Autodesk Fusion 360 part; units mm, degrees
sketch "Sketch1" plane through (0, 0, 0) normal (0, 0, 1) x (1, 0, 0)
  line L0 (-4.125, 1.2) -> (4.125, 1.2)
  line L1 (4.125, 1.2) -> (4.125, -1.2)
  line L2 (4.125, -1.2) -> (-4.125, -1.2)
  line L3 (-4.125, -1.2) -> (-4.125, 1.2)
  line L4 (-4.125, 1.2) -> (4.125, -1.2) construction
  line L5 (4.125, 1.2) -> (-4.125, -1.2) construction
  circle A0 centre (-2.925, 0) radius 1.2
  circle A1 centre (2.925, 0) radius 1.2
  line L6 (-2.925, -0.8) -> (2.925, -0.8)
  arc A2 (2.925, -0.8) -> (2.925, 0.8) centre (2.925, 0) ccw
  line L7 (2.925, 0.8) -> (-2.925, 0.8)
  arc A3 (-2.925, 0.8) -> (-2.925, -0.8) centre (-2.925, 0) ccw
  line L8 (-2.925, 0) -> (2.925, 0) construction
  dimension "d1" = 8.25
  dimension "d2" = 2.4
  dimension "d3" = 0.4
extrude "Extrude1" add sketch "Sketch1" along normal blind 6.7 contours L0 A0 A1 L7 | A0 L6 L7 A3 | A1 L6 A2 L7 | L2 A0 A1 L6 picked at (-3.9868, -0.0769) picked at (3.9868, -0.0769)
sketch "Sketch2" plane through (0, 0, 6.7) normal (0, 0, 1) x (-1, 0, 0)
  arc A0 (2.925, -0.8) -> (2.925, 0.8) centre (2.925, 0) ccw
  line L0 (2.925, -0.8) -> (-2.925, -0.8)
  arc A1 (-2.925, 0.8) -> (-2.925, -0.8) centre (-2.925, 0) ccw
  line L1 (-2.925, 0.8) -> (2.925, 0.8)
  arc A2 (2.925, -1.2) -> (2.925, 1.2) centre (2.925, 0) ccw
  line L2 (2.925, 1.2) -> (-2.925, 1.2)
  arc A3 (-2.925, 1.2) -> (-2.925, -1.2) centre (-2.925, 0) ccw
  line L3 (-2.925, -1.2) -> (2.925, -1.2)
  line L4 (2.25, 3.5) -> (-2.25, 3.5)
  arc A4 (-2.25, 3.5) -> (-2.25, -3.5) centre (-2.25, 0) ccw
  line L5 (-2.25, -3.5) -> (2.25, -3.5)
  arc A5 (2.25, -3.5) -> (2.25, 3.5) centre (2.25, 0) ccw
  line L6 (2.25, 0) -> (-2.25, 0) construction
  line L7 (5.75, 0) -> (5.75, -5.6994) construction
  line L8 (-5.75, 0) -> (-5.75, -5.542) construction
  dimension "d7" = 7
  dimension "d8" = 11.5
extrude "Extrude2" add sketch "Sketch2" along normal blind 15.3 contours A0 L0 A1 L1 | A2 L2 A3 L3 | L4 A4 L5 A5
ref_plane "WorkPlane2" through (0, 0, 28.7) normal (0, 0, -1) x (1, 0, 0)
sketch "Sketch3" plane through (0, 0, 28.7) normal (0, 0, -1) x (-1, 0, 0)
  circle A0 centre (0, 0) radius 3.2
  dimension "d12" = 6.4
loft "Loft1" add profiles "Sketch3" section 1 face at (-0.75, 1.1667, 22) section 2
extrude "Extrude3" add sketch "Sketch3" against normal blind 6.3
fillet "Fillet1" radius 20 4 edges at (0.3491, 3.1809, 28.7) (3.1809, -0.3491, 28.7) (-0.3491, -3.1809, 28.7) (-3.1809, 0.3491, 28.7)
fillet "Fillet3" radius 3 4 edges at (0, 3.5, 22) (-5.75, 0, 22) (0, -3.5, 22) (5.75, 0, 22)
sketch "Sketch4" plane through (0, 0, 35) normal (0, 0, 1) x (-1, 0, 0)
  circle A0 centre (0, 0) radius 3.2
  circle A1 centre (0, 0) radius 2.25
  dimension "d23" = 4.5
extrude "Extrude4" add sketch "Sketch4" along normal blind 20 contours A1
Geometry check sheet. Reference: the model listing, model coordinates, mm. A direction names the side the tool comes from. Give positions to 0.01 mm unless a question says otherwise; leave off trailing zeros. Write each loop counter-clockwise with the first axis right and the second up, starting at its lowest first coordinate (ties: lowest second). Pieces come first, ordered by that corner, then holes.
1) Section check B-B, the plane z = 19. Record the boundary of the cut face in (x, y), and give its area (3 significant figures).
2) Section check A-A, the plane z = 33.5. Record the boundary of the cut face in (x, y).
3) Material ranges on L1, parallel to Z at x = -1, y = 3; L2, parallel to X at y = -0.25, z = 15.5; L3, parallel to X at y = 0, z = 36, recorded low to high.
4) Release check for a two-part mould opening along Y. For faces 1 (the flat face through (0, -0.8, 3)), 2 (the flat face through (0, -1.2, 3)), 3 (the flat face through (0, 0, 55)), 4 (the flat face through (0, 0.8, 3)) record: pulls with the +Y half, pulls with the -Y half, needs draft (parallel to the pull), parting line crosses it, or undercut.
5) Gauge pin test, flat ends, axial feed: pin 1 (4.5 mm diameter, centred on x = 1, z = 3.5, fed in from -Y); pin 2 (4.5 mm diameter, centred on x = -0.5, z = 3, fed in from +Y); pin 3 (4 mm diameter, centred on x = -3.5, z = 31.5, fed in from -Y). Record the tip position at first contact, or that the pin passes through.
6) Access from +Z, -Z, +X, -X, +Y, -Y to the whole of each face (thin tool, end or side, straight path). Record for faces 5 (the cylindrical face through (-4.125, -0.026, 3.303)), 6 (the flat face through (-1.4, -2.1, 35)), 7 (the cylindrical face through (-3.725, -0.018, 3.303)).
Computed:
1. outline: (-2.25, -3.5) - (2.25, -3.5) arc R3.5 ccw to (2.25, 3.5) - (-2.25, 3.5) arc R3.5 ccw to start
1. area: 70.0 mm2
2. outline: circle Ø6.4 at (0, 0)
3. L1: z = 6.7 to 35
3. L2: x = -5.74 to 5.74
3. L3: x = -2.25 to 2.25
4. face 1: undercut
4. face 2: pulls with the -Y half
4. face 3: needs draft
4. face 4: undercut
5. pin 1: stops at y = -1.2
5. pin 2: stops at y = 1.2
5. pin 3: stops at y = -2.83
6. face 5: -Z, -X
6. face 6: +Z
6. face 7: -Z
